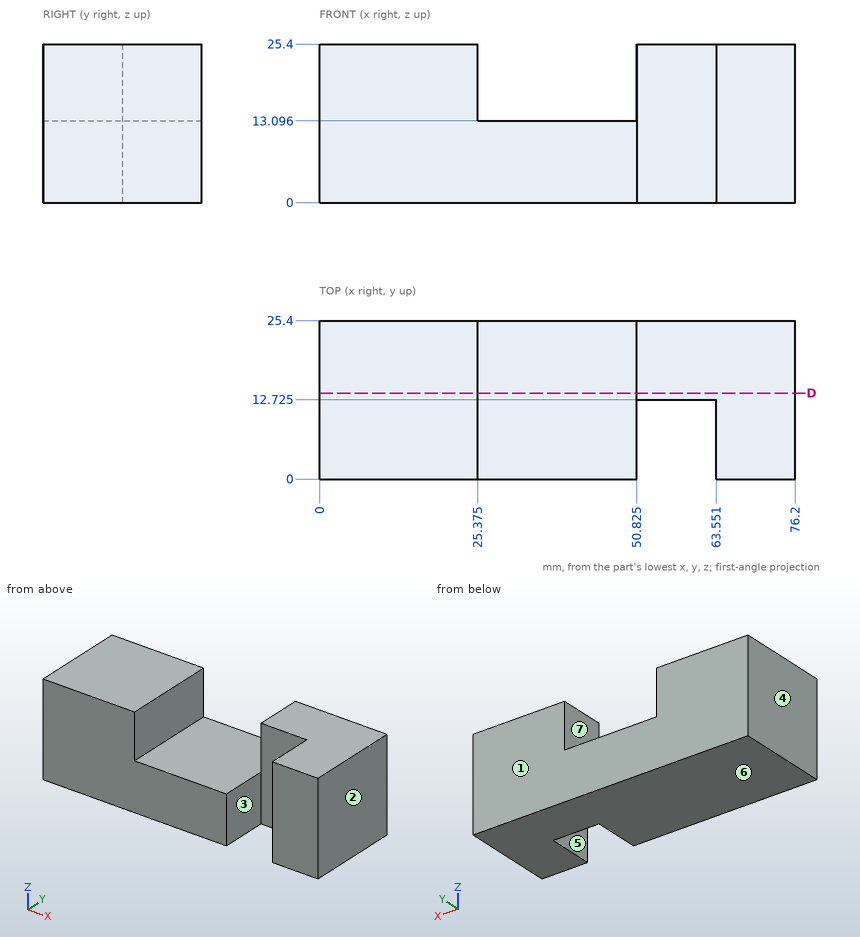
Job drawing, mm, ordinate dimensions from the low corner. One solid piece. A direction names the side the tool comes from. Round coordinates to 2 decimals unless told otherwise and drop trailing zeros. Write each loop counter-clockwise with the first axis right and the second up, starting at its lowest first coordinate (ties: lowest second). Pieces come first, ordered by that corner, then holes. Notation, with made-up numbers: M -31,1 L -21,1 A13 ccw -21,22 Z; hole C 53.25,68 d8. An arc over 180 degrees is marked long. Return JSON: item names as keys, results as strings. Group by question number.
(1) Two-plate mould, pull along X, no slides. Class the marked faces 1, 2, 3 and 4: +X half, -X half, draft (parallel to the pull), parting line (faces both ways), or undercut.
(2) Which spindle directions (+Z, -Z, +X, -X, +Y, -Y) get a long thin tool onto all of the face, cutting with end or side? Do the marked faces 5, 6 and 7. Say none if no direction does.
(3) Saw through at D-D on y = 13.75. Write the cut outline in (x, z) (1 decimal), then the cut area to 3 significant figures.
(4) Drill centre lines: probe 1 along X at (y, z) = (17.5, 23.5) (1 decimal); probe 2 along Z at (x, y) = (42.5, 18.25) (1 decimal); probe 3 along Y at (x, z) = (58, 2.5) (1 decimal). Where is each one in solid material? Low to high.
Returned:
{
 "1": {"face 1": "draft", "face 2": "+X half", "face 3": "undercut", "face 4": "-X half"},
 "2": {"face 5": "+Z, -Z, -Y", "face 6": "-Z, +X, -X, +Y, -Y", "face 7": "+Z, +Y, -Y"},
 "3": {"outline": "M 0,0 L 76.2,0 L 76.2,25.4 L 50.8,25.4 L 50.8,13.1 L 25.4,13.1 L 25.4,25.4 L 0,25.4 Z", "area": "1,620 mm²"},
 "4": {"probe 1": "0 to 25.4, 50.8 to 76.2", "probe 2": "0 to 13.1", "probe 3": "12.7 to 25.4"}
}
